Geometry: final body of the model. Coordinates: model frame, mm. A direction names the side the tool comes from. Give positions to 0.01 mm unless a question says otherwise; leave off trailing zeros. Loops run counter-clockwise (first coordinate to the right, second up) from the corner with the lowest first, then second, coordinate; pieces in that order, holes last. Notation, with made-up numbers: (-33.75, 31.25) - (-2.75, 31.25) arc R9 ccw to (-2.75, 36.25) - close; hole circle Ø9 at (59, 51). An arc over 180 degrees is marked (long way). Answer in a Markdown table with one row per item.
Autodesk Inventor part; units mm, degrees
ref_plane "Arbeitsebene1" through (-20.2254, 10, 14.6946) normal (-0.809017, 0, 0.5877853) x (0, -1, 0)
ref_plane "Arbeitsebene2" through (25, 0, 0) normal (1, 0, 0) x (0, 1, 0)
ref_plane "YZ Plane" through (0, 0, 0) normal (1, 0, 0) x (0, 1, 0)
sketch "Skizze1" plane through (0, 0, 0) normal (0, 1, 0) x (-1, 0, 0)
  circle A0 centre (0, 0) radius 7.5
  circle A1 centre (0, 0) radius 25
  dimension "d0" = 15
  dimension "d1" = 50
extrude "Extrusion1" add sketch "Skizze1" along normal blind 10
sketch "Skizze2" plane through (0, 10, 0) normal (0, 1, 0) x (1, 0, 0)
  circle A0 centre (0, 0) radius 25
  line L0 (-25, 0) -> (-16.25, 0)
  line L1 (0, 0) -> (8.75, 0) construction
  line L2 (0, 0) -> (-5.0215, 15.4547)
  line L3 (0, 0) -> (16.25, 0) construction
  line L4 (0, 0) -> (13.1465, 9.5515)
  line L5 (0, 0) -> (16.25, 0) construction
  line L6 (0, 0) -> (16.25, 0) construction
  line L7 (0, 0) -> (13.1465, -9.5515)
  line L8 (0, 0) -> (16.25, 0) construction
  line L9 (0, 0) -> (-5.0215, -15.4547)
  line L10 (0, 0) -> (16.25, 0) construction
  circle A1 centre (-16.25, 0) radius 4.3
  circle A2 centre (-5.0215, 15.4547) radius 4.3
  circle A3 centre (13.1465, 9.5515) radius 4.3
  circle A4 centre (13.1465, -9.5515) radius 4.3
  circle A5 centre (-5.0215, -15.4547) radius 4.3
  dimension "d4" = 8.75
  dimension "d9" = 16.25
  dimension "d10" = 108
  dimension "d11" = 16.25
  dimension "d12" = 36
  dimension "d15" = 16.25
  dimension "d16" = 36
  dimension "d17" = 16.25
  dimension "d18" = 108
  dimension "d19" = 8.6
  dimension "d20" = 8.6
  dimension "d21" = 8.6
  dimension "d22" = 8.6
  dimension "d23" = 8.6
hole "Bohrung1" at (-16.25, 10, 0) at (-5.0215, 10, -15.4547) at (13.1465, 10, -9.5515) at (13.1465, 10, 9.5515) at (-5.0215, 10, 15.4547) direction (0, -1, 0) diameter 9 end through all
sketch "Skizze3" plane through (0, 0, 0) normal (1, 0, 0) x (0, 1, 0)
  point P0 (0, 0)
sketch "Skizze4" plane through (0, 0, 0) normal (1, 0, 0) x (0, 1, 0)
  line L0 (0, 0) -> (5, 0)
sketch "Skizze6" plane through (0, 10, 0) normal (0, 1, 0) x (1, 0, 0)
  circle A0 centre (-5.0215, -15.4547) radius 4.5
  circle A1 centre (-16.25, 0) radius 4.5
  circle A2 centre (0, 0) radius 25
  line L0 (0, 0) -> (-8.7488, -12.9333)
  line L1 (0, 0) -> (-15.0038, -4.324)
  line L2 (-11.8428, -8.6043) -> (-20.2254, -14.6946)
  line L3 (-11.8428, -8.6043) -> (-1.4813, -8.6043) construction
  line L4 (0, 0) -> (-11.8428, -8.6043)
  dimension "d36" = 5.321
  dimension "d37" = 144
sketch "Skizze7" plane through (0, 0, 0) normal (0, -1, 0) x (1, 0, 0)
  line L0 (0, 0) -> (-20.2254, 14.6946)
  circle A0 centre (0, 0) radius 25
  line L1 (0, 0) -> (25, 0) construction
  line L2 (-20.2254, 14.6946) -> (44.6167, -28.5072)
  dimension "d38" = 144
ref_plane "Arbeitsebene1" through (-20.2254, 10, 14.6946) normal (-0.809017, 0, 0.5877853) x (0, -1, 0)
sketch "Skizze8" plane through (-20.2254, 10, 14.6946) normal (-0.809017, 0, 0.5877853) x (0, -1, 0)
  line L0 (10, 0) -> (5, 0)
  dimension "d39" = 5
hole "Bohrung2" at (-20.2254, 5, 14.6946) direction (0.809017, 0, -0.5877853) diameter 2.459 depth 27.8 tip angle 118
sketch "Skizze9" plane through (0, 0, 0) normal (0, -1, 0) x (1, 0, 0)
  line L0 (0, 0) -> (25, 0)
  circle A0 centre (0, 0) radius 25
  line L1 (0, 0) -> (14.68, 5.3208)
  circle A1 centre (13.1465, 9.5515) radius 4.5
  line L2 (0, 0) -> (14.68, -5.3208)
  circle A2 centre (13.1465, -9.5515) radius 4.5
  line L3 (0, 0) -> (25, 0)
sketch "Skizze10" plane through (0, 10, 0) normal (0, 1, 0) x (1, 0, 0)
  line L0 (0, 0) -> (25, 0)
  circle A0 centre (0, 0) radius 25
ref_plane "Arbeitsebene2" through (25, 0, 0) normal (1, 0, 0) x (0, 1, 0)
sketch "Skizze11" plane through (25, 0, 0) normal (1, 0, 0) x (0, 1, 0)
  line L0 (0, 0) -> (5, 0)
  dimension "d47" = 5
hole "Bohrung3" at (25, 5, 0) direction (-1, 0, 0) diameter 2.459 depth 27.8 tip angle 118
properties part number "Flansch" material "Aluminium 6061"
Q1. Cut plane D-D (z = -15). Output: boundary loops of the cut face in (x, y), and give its area (3 significant figures).
Check values:
| item | result |
|---|---|
| outline | (-20, 0) - (-9.5, 0) - (-9.5, 10) - (-20, 10) - close; (-0.54, 0) - (20, 0) - (20, 10) - (-0.54, 10) - close |
| area | 310 mm² |
Q2. First-contact query: pin 1 (1.5 mm diameter, centred on x = -0.5, y = 7, fed in from +Z); pin 2 (5 mm diameter, centred on y = 8, z = 3, fed in from +X) (3 decimals); pin 3 (1.5 mm diameter, centred on y = 6, z = -16, fed in from -X). Flat tips, straight axial feed; report the tip coordinate or a pass-through.
Check values:
| item | result |
|---|---|
| pin 1 | z = 25 |
| pin 2 | x = 24.995 |
| pin 3 | x = -19.81 |
Q3. Draft query along Z for faces 1 (the cylindrical face through (-2.283, 4.93, 11.884)), 2 (the flat face through (-5, 0, 6)), 3 (the cylindrical face through (-23.846, 4.93, -7.509)). Return one class per face: pulls with the +Z half, pulls with the -Z half, needs draft (parallel to the pull), parting line crosses it, or undercut.
Check values:
| item | result |
|---|---|
| face 1 | undercut |
| face 2 | needs draft |
| face 3 | parting line crosses it |
Q4. Cut plane B-B (x = 16). Output: boundary loops of the cut face in (y, z).
Check values:
| item | result |
|---|---|
| outline | (0, -19.21) - (10, -19.21) - (10, -13.03) - (0, -13.03) - close; (0, -6.07) - (10, -6.07) - (10, 6.07) - (0, 6.07) - close; (0, 13.03) - (10, 13.03) - (10, 19.21) - (0, 19.21) - close; hole circle Ø2.46 at (5, 0) |
Q5. Material intervals for line 1 along X through (y, z) = (3.25, 0); line 2 along X through (y, z) = (4, -4); line 3 along X through (y, z) = (4.5, 0), sorted ascending.
Check values:
| item | result |
|---|---|
| line 1 | -25 to -20.75, -11.75 to -7.5, 7.5 to 25 |
| line 2 | -24.68 to -18.31, -14.19 to -6.34, 6.34 to 24.68 |
| line 3 | -25 to -20.75, -11.75 to -7.5 |
Q6. Reachability of faces 4 (the cylindrical face through (16.08, 6.09, -0.57)), 5 (the cylindrical face through (-20.71, 4.93, -0.59)) from +Z, -Z, +X, -X, +Y, -Y: full face, straight path, thin tool, end or side. Return the list, or none.
Check values:
| item | result |
|---|---|
| face 4 | +X |
| face 5 | +Y, -Y |
Q7. Cut plane A-A (z = 0). Output: boundary loops of the cut face in (x, y), and give its area (3 significant figures).
Check values:
| item | result |
|---|---|
| outline | (-25, 0) - (-20.75, 0) - (-20.75, 10) - (-25, 10) - close; (-11.75, 0) - (-7.5, 0) - (-7.5, 10) - (-11.75, 10) - close; (7.5, 0) - (25, 0) - (25, 3.77) - (7.5, 3.77) - close; (7.5, 6.23) - (25, 6.23) - (25, 10) - (7.5, 10) - close |
| area | 217 mm² |
Q8. Cut plane C-C (y = 5). Output: boundary loops of the cut face in (x, z).
Check values:
| item | result |
|---|---|
| outline | (-20.92, 13.68) arc R25 ccw (long way) to (24.97, -1.23) - (7.4, -1.23) arc R7.5 cw (long way) to (-6.71, 3.35) - close; (-19.48, 15.67) - (-5.26, 5.34) arc R7.5 cw to (7.4, 1.23) - (24.97, 1.23) arc R25 ccw to start; hole circle Ø9 at (-16.25, 0); hole circle Ø9 at (-5.02, -15.45); hole circle Ø9 at (-5.02, 15.45); hole circle Ø9 at (13.15, -9.55); hole circle Ø9 at (13.15, 9.55) |
